Part model, mm, in its own coordinate system. A direction names the side the tool comes from. Round coordinates to 2 decimals unless told otherwise and drop trailing zeros. Loops run counter-clockwise (first coordinate to the right, second up) from the corner with the lowest first, then second, coordinate; pieces in that order, holes last. Notation, with made-up numbers: (60.25, -27.75) - (65.25, -27.75) arc R24 cw to (65.25, 0.25) - close; hole circle Ø6 at (29, -33). An arc over 180 degrees is marked (long way). Write each question's results on one line, items separated by ' | '. Start each with the question number.
(1) Drill centre lines: L1, parallel to Y at x = 0, z = 0.95; L2, parallel to Y at x = -4.5, z = 2.9; L3, parallel to X at y = 2, z = 0.8. Where is each one in solid material? Low to high.
(2) Tool access for faces 5 (the face through (-17, 30.041, 2)), 6 (the face through (2.041, -32, 2)), 7 (the face through (9.459, 32, 2)), 8 (the face through (13.541, 32, 2)), 9 (the face through (-17, -30.041, 2)): list every direction of +Z, -Z, +X, -X, +Y, -Y with a clear straight run to the whole face (end or side of a thin tool).
(3) Flat gauge pins, fed straight in: P1, Ø1, axis at x = 6.5, z = 1, coming from the -Y side; P2, Ø1, axis at y = -32.5, z = 1, coming from the +X side; P3, Ø1.6, axis at y = -31, z = 1, coming from the -X side; P4, Ø6, axis at x = -9, y = 14.5, coming from the -Z side. Where does each tip first touch, or does it go through?
(4) Cut at B-B, the plane x = 0. List the corners of the cut face in (y, z) (3 decimals), then the cut area to 3 significant figures.
(5) Cut at A-A, the plane y = 0. List the corners of the cut face in (x, z) (3 decimals).
(6) Mould opens along X. For faces 1 (the face through (-11, 33.216, 2)), 2 (the face through (21.191, 0, 2)), 3 (the face through (-9.459, 32, 2)), 4 (the face through (-1.73, -7.77, 1.61)) say: released by +X, released by -X, zero draft, split by the parting line, or undercut.
(7) Cut at D-D, the plane x = 16. List the corners of the cut face in (y, z) (3 decimals), then the cut area to 3 significant figures.
from build123d import *

# Parameters (mm, degrees)
SKETCH1_R           = 8
BOSS_EXTRUDE1_DEPTH = 3.175
SKETCH2_R           = 7.95936
BOSS_EXTRUDE3_DEPTH = 3.175


with BuildPart() as part:
    # Sketch1 → Boss-Extrude1 (new body)
    with BuildSketch(Plane.XY):
        Polygon((-13.5, 30), (-21.15, 30), (-21.15, -30), (-13.5, -30), (-13.5, -33.175), (-9.5, -33.175), (-9.5, -30), (-2, -30), (-2, -33.175), (2, -33.175), (2, -30), (9.5, -30), (9.5, -33.175), (13.5, -33.175), (13.5, -30), (21.15, -30), (21.15, 30), (13.5, 30), (13.5, 33.175), (9.5, 33.175), (9.5, 30), (2, 30), (2, 33.175), (-2, 33.175), (-2, 30), (-9.5, 30), (-9.5, 33.175), (-13.5, 33.175), align=None)
        Circle(SKETCH1_R, mode=Mode.SUBTRACT)
    extrude(amount=BOSS_EXTRUDE1_DEPTH)

    # Sketch2 → Boss-Extrude3 (add)
    with BuildSketch(Plane.XY.offset(3.175)):
        Polygon((21.19064, -30.04064), (21.19064, 30.04064), (13.54064, 30.04064), (13.54064, 33.21564), (9.45936, 33.21564), (9.45936, 30.04064), (2.04064, 30.04064), (2.04064, 33.21564), (-2.04064, 33.21564), (-2.04064, 30.04064), (-9.45936, 30.04064), (-9.45936, 33.21564), (-13.54064, 33.21564), (-13.54064, 30.04064), (-21.19064, 30.04064), (-21.19064, -30.04064), (-13.54064, -30.04064), (-13.54064, -33.21564), (-9.45936, -33.21564), (-9.45936, -30.04064), (-2.04064, -30.04064), (-2.04064, -33.21564), (2.04064, -33.21564), (2.04064, -30.04064), (9.45936, -30.04064), (9.45936, -33.21564), (13.54064, -33.21564), (13.54064, -30.04064), align=None)
        Circle(SKETCH2_R, mode=Mode.SUBTRACT)
    extrude(amount=-BOSS_EXTRUDE3_DEPTH)


solid = part.part
A:
1) L1: -33.22 to -7.96, 7.96 to 33.22 | L2: -30.04 to -6.57, 6.57 to 30.04 | L3: -21.19 to -7.7, 7.7 to 21.19
2) face 5: +Z, -Z, -X, +Y | face 6: +Z, -Z, -Y | face 7: +Z, -Z, +Y | face 8: +Z, -Z, +X, +Y | face 9: +Z, -Z, -X, -Y
3) P1: y = -30.04 | P2: x = 13.54 | P3: x = -13.54 | P4: z = 0
4) outline: (-33.216, 0) - (-7.959, 0) - (-7.959, 3.175) - (-33.216, 3.175) - close; (7.959, 0) - (33.216, 0) - (33.216, 3.175) - (7.959, 3.175) - close | area: 160 mm2
5) outline: (-21.191, 0) - (-7.959, 0) - (-7.959, 3.175) - (-21.191, 3.175) - close; (7.959, 0) - (21.191, 0) - (21.191, 3.175) - (7.959, 3.175) - close
6) face 1: zero draft | face 2: released by +X | face 3: undercut | face 4: undercut
7) outline: (-30.041, 0) - (30.041, 0) - (30.041, 3.175) - (-30.041, 3.175) - close | area: 191 mm2
